```python
from build123d import *

# Parameters (mm, degrees)
BOX_W             = 22
BOX_H             = 122
BOX_DEPTH         = 3
BOX001_W          = 10
BOX001_H          = 17
BOX001_DEPTH      = 3
BOX002_W          = 10
BOX002_H          = 17
BOX002_DEPTH      = 3
BOX003_W          = 46
BOX003_H          = 5.5
BOX003_DEPTH      = 5
CYLINDER002_R     = 1.5
CYLINDER002_DEPTH = 5
CYLINDER003_R     = 1.5
CYLINDER003_DEPTH = 5
BOX004_W          = 2
BOX004_H          = 30
BOX004_DEPTH      = 2
CYLINDER_R        = 1.4
CYLINDER_DEPTH    = 5
CYLINDER004_R     = 1.4
CYLINDER004_DEPTH = 5


with BuildPart() as part:
    # Box → Box (join)
    with BuildSketch(Plane(origin=(-10, -62.5, 0), x_dir=(1, 0, 0), z_dir=(0, 0, 1))):
        with Locations((11, 61)):
            Rectangle(BOX_W, BOX_H)
    extrude(amount=BOX_DEPTH)

    # Box001 → Box001 (join)
    with BuildSketch(Plane(origin=(-10, -44.5, 0), x_dir=(0, 1, 0), z_dir=(1, 0, 0))):
        with Locations((5, 8.5)):
            Rectangle(BOX001_W, BOX001_H)
    extrude(amount=BOX001_DEPTH)

    # Box002 → Box002 (join)
    with BuildSketch(Plane(origin=(-10, 24.5, 0), x_dir=(0, 1, 0), z_dir=(1, 0, 0))):
        with Locations((5, 8.5)):
            Rectangle(BOX002_W, BOX002_H)
    extrude(amount=BOX002_DEPTH)

    # Box003 → Box003 (cut)
    with BuildSketch(Plane(origin=(-3.5, 19.5, -1), x_dir=(0, -1, 0), z_dir=(0, 0, 1))):
        with Locations((23, 2.75)):
            Rectangle(BOX003_W, BOX003_H)
    extrude(amount=BOX003_DEPTH, mode=Mode.SUBTRACT)

    # Cylinder002 → Cylinder002 (cut)
    with BuildSketch(Plane(origin=(0.8, -59, -1), x_dir=(0, 1, 0), z_dir=(0, 0, 1))):
        Circle(CYLINDER002_R)
    extrude(amount=CYLINDER002_DEPTH, mode=Mode.SUBTRACT)

    # Cylinder003 → Cylinder003 (cut)
    with BuildSketch(Plane(origin=(0.8, 56, -1), x_dir=(0, 1, 0), z_dir=(0, 0, 1))):
        Circle(CYLINDER003_R)
    extrude(amount=CYLINDER003_DEPTH, mode=Mode.SUBTRACT)

    # Box004 → Box004 (cut)
    with BuildSketch(Plane(origin=(16.8, -62.5, -1), x_dir=(0, 1, 0), z_dir=(0, 0, 1))):
        with Locations((1, 15)):
            Rectangle(BOX004_W, BOX004_H)
    extrude(amount=BOX004_DEPTH, mode=Mode.SUBTRACT)

    # Cylinder → Cylinder (cut)
    with BuildSketch(Plane(origin=(-6, -40.5, 10), x_dir=(0, -1, 0), z_dir=(-1, 0, 0))):
        Circle(CYLINDER_R)
    extrude(amount=CYLINDER_DEPTH, mode=Mode.SUBTRACT)

    # Cylinder004 → Cylinder004 (cut)
    with BuildSketch(Plane(origin=(-6, 29, 10), x_dir=(0, -1, 0), z_dir=(-1, 0, 0))):
        Circle(CYLINDER004_R)
    extrude(amount=CYLINDER004_DEPTH, mode=Mode.SUBTRACT)


solid = part.part
```
The listing builds one solid part. Answer for the finished solid, in the listing's coordinates (mm). A direction names the side the tool comes from. Give positions to 0.01 mm unless a question says otherwise; leave off trailing zeros. Order: outer loops, then holes, each group sorted by start corner. A loop starts at its lowest first (then second) coordinate and runs counter-clockwise, first axis right, second up. Notation, with made-up numbers: (-23, -13) - (16, -13) arc R7 cw to (16, -7) - close; hole circle Ø11 at (54.25, 75). An arc over 180 degrees is marked (long way). Answer in a Markdown table with one row per item. Add a question column.
Q1. The part is cut by section A-A (y = -40.5). Determine the outline of the cut face in (x, z).
Q2. For a pull along Z with two mould halves and no side action, classify faces 1 (the flat face through (-1, 19.5, 1)), 2 (the flat face through (-9, -40, 17)), 3 (the cylindrical face through (-8.479, -41.835, 10.421)) as released by +Z, released by -Z, zero draft, split by the parting line, or undercut.
Q3. The part is cut by section B-B (z = 15). Determine the outline of the cut face in (x, y).
Q4. The part is cut by section D-D (y = -5.5). Determine the outline of the cut face in (x, z).
Q5. Find the intervals of material crossed by line 1 along Y through (x, z) = (-9, 10); line 2 along X through (y, z) = (56, 1); line 3 along Z through (x, y) = (-7.25, -6), in increasing order. Write a range as [from, to].
Q6. The part is cut by section C-C (z = 10). Determine the outline of the cut face in (x, y).
Q7. Which of the six approach directions +Z, -Z, +X, -X, +Y, -Y give full straight-line access (tool end or side, diameter ignored) to faces 4 (the flat face through (-9, 24.5, 10)), 5 (the flat face through (1, -62, 1)), 6 (the flat face through (-1, -26.5, 1)), 7 (the flat face through (-9, -44.5, 10))?
Q8. Given P1, Ø1.6, axis at x = -1.5, y = -61.5, coming from the -Z side; P2, Ø4, axis at x = 2.5, y = 10.5, coming from the +Z side; P3, Ø0.9, axis at x = -8, z = 13, coming from the -Y side, each flat-ended and moving along its own axis, determine where each tip first touches the part or whether it passes through.
Determined:
| question | item | result |
|---|---|---|
| 1 | outline | (-10, 0) - (12, 0) - (12, 3) - (-7, 3) - (-7, 8.6) - (-10, 8.6) - close; (-10, 11.4) - (-7, 11.4) - (-7, 17) - (-10, 17) - close |
| 2 | face 1 | zero draft |
| 2 | face 2 | released by +Z |
| 2 | face 3 | undercut |
| 3 | outline | (-10, -44.5) - (-7, -44.5) - (-7, -34.5) - (-10, -34.5) - close; (-10, 24.5) - (-7, 24.5) - (-7, 34.5) - (-10, 34.5) - close |
| 4 | outline | (-10, 0) - (-3.5, 0) - (-3.5, 3) - (-10, 3) - close; (2, 0) - (12, 0) - (12, 3) - (2, 3) - close |
| 5 | line 1 | y = [-44.5, -41.9], [-39.1, -34.5], [24.5, 27.6], [30.4, 34.5] |
| 5 | line 2 | x = [-10, -0.7], [2.3, 12] |
| 5 | line 3 | z = [0, 3] |
| 6 | outline | (-10, -44.5) - (-7, -44.5) - (-7, -41.9) - (-10, -41.9) - close; (-10, -39.1) - (-7, -39.1) - (-7, -34.5) - (-10, -34.5) - close; (-10, 24.5) - (-7, 24.5) - (-7, 27.6) - (-10, 27.6) - close; (-10, 30.4) - (-7, 30.4) - (-7, 34.5) - (-10, 34.5) - close |
| 7 | face 4 | +Z, +X, -X |
| 7 | face 5 | -Z, +X, -X, -Y |
| 7 | face 6 | +Z, -Z |
| 7 | face 7 | +Z, +X, -X, -Y |
| 8 | P1 | stops at z = 1 |
| 8 | P2 | stops at z = 3 |
| 8 | P3 | stops at y = -44.5 |
